Design review of the part built by this model. Coordinates are the model's own, in mm. A direction names the side the tool comes from. Coordinates: 2 decimals unless noted, no trailing zeros. Order: outer loops, then holes, each group sorted by start corner. A loop starts at its lowest first (then second) coordinate and runs counter-clockwise, first axis right, second up. Notation, with made-up numbers: M 70.25,-13 L 74.25,-13 A24 ccw 74.25,23 Z; hole C 8.5,30.5 d5. An arc over 180 degrees is marked long. Answer in a Markdown table with one row per item.
from build123d import *

# Parameters (mm, degrees)
SKETCH2_W           = 210
SKETCH2_H           = 105
SKETCH2_W_2         = 190
SKETCH2_H_2         = 50
BOSS_EXTRUDE2_DEPTH = 150
FILLET1_R           = 10
FILLET2_R           = 10
FILLET3_R           = 10
FILLET4_R           = 10
SKETCH3_R           = 16.1
CUT_EXTRUDE1_DEPTH  = 10
SKETCH4_W           = 230
SKETCH4_H           = 125
BOSS_EXTRUDE3_DEPTH = 10
FILLET5_R           = 10
FILLET6_R           = 10
FILLET7_R           = 10
FILLET8_R           = 10
SKETCH7_W           = 10
SKETCH7_H           = 50
BOSS_EXTRUDE4_DEPTH = 75
SKETCH8_R           = 16.1
CUT_EXTRUDE2_DEPTH  = 10


with BuildPart() as part:
    # Sketch2 → Boss-Extrude2 (new body)
    with BuildSketch(Plane(origin=(0, 0, 0), x_dir=(1, 0, 0), z_dir=(0, 1, 0))):
        Rectangle(SKETCH2_W, SKETCH2_H)
        Rectangle(SKETCH2_W_2, SKETCH2_H_2, mode=Mode.SUBTRACT)
    extrude(amount=BOSS_EXTRUDE2_DEPTH)

    # Fillet1
    fillet1_edges = [part.edges().sort_by_distance(p)[0] for p in [
        (-105, 75, -52.5),
    ]]
    fillet(fillet1_edges, radius=FILLET1_R)

    # Fillet2
    fillet2_edges = [part.edges().sort_by_distance(p)[0] for p in [
        (-105, 75, 52.5),
    ]]
    fillet(fillet2_edges, radius=FILLET2_R)

    # Fillet3
    fillet3_edges = [part.edges().sort_by_distance(p)[0] for p in [
        (105, 75, 52.5),
    ]]
    fillet(fillet3_edges, radius=FILLET3_R)

    # Fillet4
    fillet4_edges = [part.edges().sort_by_distance(p)[0] for p in [
        (105, 75, -52.5),
    ]]
    fillet(fillet4_edges, radius=FILLET4_R)

    # Sketch3 → Cut-Extrude1 (cut)
    with BuildSketch(Plane.ZY.offset(105)):
        with Locations((0, 75)):
            Circle(SKETCH3_R)
    extrude(amount=-CUT_EXTRUDE1_DEPTH, mode=Mode.SUBTRACT)

    # Sketch4 → Boss-Extrude3 (add)
    with BuildSketch(Plane(origin=(0, 0, 0), x_dir=(1, 0, 0), z_dir=(0, 1, 0))):
        Rectangle(SKETCH4_W, SKETCH4_H)
    extrude(amount=-BOSS_EXTRUDE3_DEPTH)

    # Fillet5
    fillet5_edges = [part.edges().sort_by_distance(p)[0] for p in [
        (115, -5, 62.5),
    ]]
    fillet(fillet5_edges, radius=FILLET5_R)

    # Fillet6
    fillet6_edges = [part.edges().sort_by_distance(p)[0] for p in [
        (115, -5, -62.5),
    ]]
    fillet(fillet6_edges, radius=FILLET6_R)

    # Fillet7
    fillet7_edges = [part.edges().sort_by_distance(p)[0] for p in [
        (-115, -5, -62.5),
    ]]
    fillet(fillet7_edges, radius=FILLET7_R)

    # Fillet8
    fillet8_edges = [part.edges().sort_by_distance(p)[0] for p in [
        (-115, -5, 62.5),
    ]]
    fillet(fillet8_edges, radius=FILLET8_R)

    # Sketch7 → Boss-Extrude4 (add)
    with BuildSketch(Plane(origin=(0, 0, 0), x_dir=(1, 0, 0), z_dir=(0, 1, 0))):
        Rectangle(SKETCH7_W, SKETCH7_H)
    extrude(amount=BOSS_EXTRUDE4_DEPTH)

    # Sketch8 → Cut-Extrude2 (cut)
    with BuildSketch(Plane.ZY.offset(5)):
        with Locations((0, 75)):
            Circle(SKETCH8_R)
    extrude(amount=-CUT_EXTRUDE2_DEPTH, mode=Mode.SUBTRACT)


solid = part.part
(1) Add section B-B, the plane y = 36.5. Give the boundary of the cut face in (x, z).
Return value:
| item | result |
|---|---|
| outline | M -105,-42.5 A10 ccw -95,-52.5 L 95,-52.5 A10 ccw 105,-42.5 L 105,42.5 A10 ccw 95,52.5 L -95,52.5 A10 ccw -105,42.5 Z; hole M -95,-25 L -5,-25 L -5,25 L -95,25 Z; hole M 5,-25 L 95,-25 L 95,25 L 5,25 Z |
(2) Add section C-C, the plane z = 0. Give the boundary of the cut face in (x, y).
Return value:
| item | result |
|---|---|
| outline | M -115,-10 L 115,-10 L 115,0 L 105,0 L 105,150 L 95,150 L 95,0 L 5,0 L 5,58.9 L -5,58.9 L -5,0 L -95,0 L -95,58.9 L -105,58.9 L -105,0 L -115,0 Z; M -105,91.1 L -95,91.1 L -95,150 L -105,150 Z |
(3) For faces 1 (the cylindrical face through (-0.07, 58.904, -0.354)), 2 (the flat face through (-1, 74, -52.5)), 3 (the flat face through (-5, 37, 0)), 4 (the flat face through (105, 74, 1)), 5 (the flat face through (-105, 57, 1)), list the 3-axis set-ups (+Z, -Z, +X, -X, +Y, -Y) from which the entire face can be reached by the end or side of a thin tool; tool diameter is ignored.
Return value:
| item | result |
|---|---|
| face 1 | -X, +Y |
| face 2 | -Z, +X, -X, +Y |
| face 3 | +Y |
| face 4 | +Z, -Z, +X, +Y |
| face 5 | +Z, -Z, -X, +Y |
(4) Insertion check: pin 1 Ø10 at (y, z) = (8.5, 7) entering from -X; pin 2 Ø1 at (x, z) = (71, -5) entering from +Y; pin 3 Ø10 at (x, z) = (0.5, -20.5) entering from +Y; pin 4 Ø25 at (y, z) = (66, -11) entering from +X. Each pin has a flat end and moves straight along its axis. Give the tip position at first contact, or say it passes through.
Return value:
| item | result |
|---|---|
| pin 1 | stops at x = -105 |
| pin 2 | stops at y = 0 |
| pin 3 | stops at y = 150 |
| pin 4 | stops at x = 105 |
(5) Add section D-D, the plane x = -51.5. Give the boundary of the cut face in (y, z).
Return value:
| item | result |
|---|---|
| outline | M -10,-62.5 L 0,-62.5 L 0,-52.5 L 150,-52.5 L 150,-25 L 0,-25 L 0,25 L 150,25 L 150,52.5 L 0,52.5 L 0,62.5 L -10,62.5 Z |
(6) Add section A-A, the plane y = 107. Give the boundary of the cut face in (x, z).
Return value:
| item | result |
|---|---|
| outline | M -105,-42.5 A10 ccw -95,-52.5 L 95,-52.5 A10 ccw 105,-42.5 L 105,42.5 A10 ccw 95,52.5 L -95,52.5 A10 ccw -105,42.5 Z; hole M -95,-25 L 95,-25 L 95,25 L -95,25 Z |
(7) Draft analysis for pull direction X (two halves, no side actions). For faces 6 (the cylindrical face through (101.99, 76.05, 49.65)), 7 (the flat face through (-95, 57, 0)), 8 (the cylindrical face through (-100.07, 90.963, -2.096)), state which applies: pulls with the +X half, pulls with the -X half, needs draft (parallel to the pull), parting line crosses it, or undercut.
Return value:
| item | result |
|---|---|
| face 6 | pulls with the +X half |
| face 7 | undercut |
| face 8 | needs draft |
(8) For line 1 along X through (y, z) = (26, 7); line 2 along Y through (x, z) = (-102, 0); line 3 along Z through (x, y) = (83, 78), list the stretches that pass through material, from the lowest coordinate up. Write a range as from..to.
Return value:
| item | result |
|---|---|
| line 1 | x = -105..-95, -5..5, 95..105 |
| line 2 | y = -10..58.9, 91.1..150 |
| line 3 | z = -52.5..-25, 25..52.5 |
